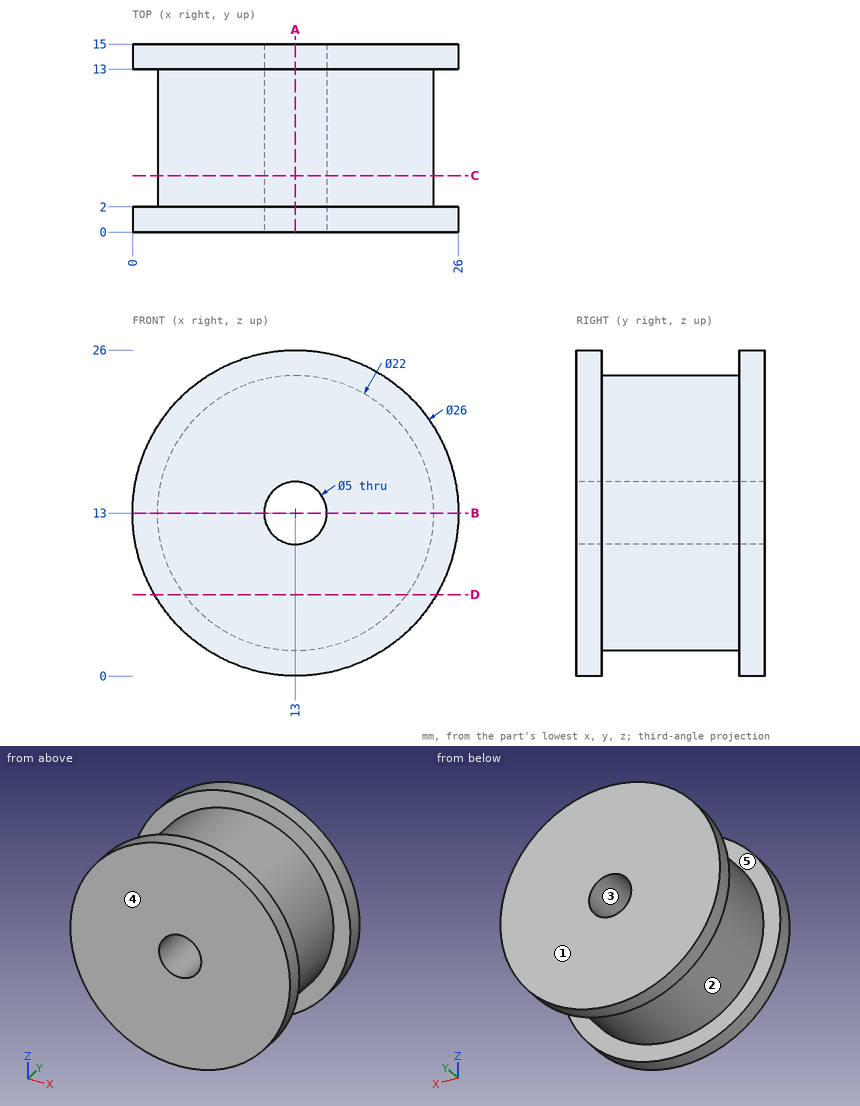
Source: three-view drawing plus pictorial views. Frame: mm from the lowest corner of the part. A direction names the side the tool comes from. Give positions to 0.01 mm unless a question says otherwise; leave off trailing zeros. Write each loop counter-clockwise with the first axis right and the second up, starting at its lowest first coordinate (ties: lowest second). Pieces come first, ordered by that corner, then holes. Notation, with made-up numbers: (32, -33) -> (62, -33) arc R24 ccw to (62, -5) -> close; hole circle Ø8 at (22.25, 82). An arc over 180 degrees is marked (long way). Write item = value, one per line.
Q1. Reachability of the marked faces 4 and 5 from +Z, -Z, +X, -X, +Y, -Y: full face, straight path, thin tool, end or side. Return the list, or none.
Here are the results:
face_4 = +Z, -Z, +X, -X, -Y
face_5 = none
Q2. Cut plane B-B on z = 13. Return loops of the section in (x, y), then the cut area to 3 significant figures.
Here are the results:
outline = (0, 0) -> (10.5, 0) -> (10.5, 15) -> (0, 15) -> (0, 13) -> (2, 13) -> (2, 2) -> (0, 2) -> close; (15.5, 0) -> (26, 0) -> (26, 2) -> (24, 2) -> (24, 13) -> (26, 13) -> (26, 15) -> (15.5, 15) -> close
area = 271 mm²
Q3. Cut plane D-D on z = 6.5. Return loops of the section in (x, y).
Here are the results:
outline = (1.74, 0) -> (24.26, 0) -> (24.26, 2) -> (21.87, 2) -> (21.87, 13) -> (24.26, 13) -> (24.26, 15) -> (1.74, 15) -> (1.74, 13) -> (4.13, 13) -> (4.13, 2) -> (1.74, 2) -> close
Q4. First-contact query: pin 1 (6 mm diameter, centred on x = 13, z = 13, fed in from +Y); pin 2 (2 mm diameter, centred on y = 6.5, z = 8, fed in from -X); pin 3 (4 mm diameter, centred on y = 11.5, z = 7, fed in from +X); pin 4 (5 mm diameter, centred on x = 2.5, y = 8, fed in from -Z). Flat tips, straight axial feed; report the tip coordinate or a pass-through.
Here are the results:
pin_1 = 15
pin_2 = 2.75
pin_3 = 25.13
pin_4 = 5.45
Q5. Line query: line 1 (X direction, y = 6.5, z = 13); line 2 (Y direction, x = 8, z = 2.5); line 3 (Z direction, x = 14, y = 11.75). Output: solid intervals per line, ascending. Write a range as from..to.
Here are the results:
line_1 = 2..10.5, 15.5..24
line_2 = 0..2, 13..15
line_3 = 2.05..10.71, 15.29..23.95
Q6. Cut plane C-C on y = 4.5. Return loops of the section in (x, z), then the cut area to 3 significant figures.
Here are the results:
outline = circle Ø22 at (13, 13); hole circle Ø5 at (13, 13)
area = 360 mm²
Q7. Mould query, pull axis X, two halves, no side actions, for the marked faces 1, 2 and 3. Classes: +X half, -X half, draft (parallel to the pull), parting line (faces both ways), or undercut.
Here are the results:
face_1 = draft
face_2 = parting line
face_3 = undercut
Q8. Cut plane A-A on x = 13. Return loops of the section in (y, z), then the cut area to 3 significant figures.
Here are the results:
outline = (0, 0) -> (2, 0) -> (2, 2) -> (13, 2) -> (13, 0) -> (15, 0) -> (15, 10.5) -> (0, 10.5) -> close; (0, 15.5) -> (15, 15.5) -> (15, 26) -> (13, 26) -> (13, 24) -> (2, 24) -> (2, 26) -> (0, 26) -> close
area = 271 mm²
